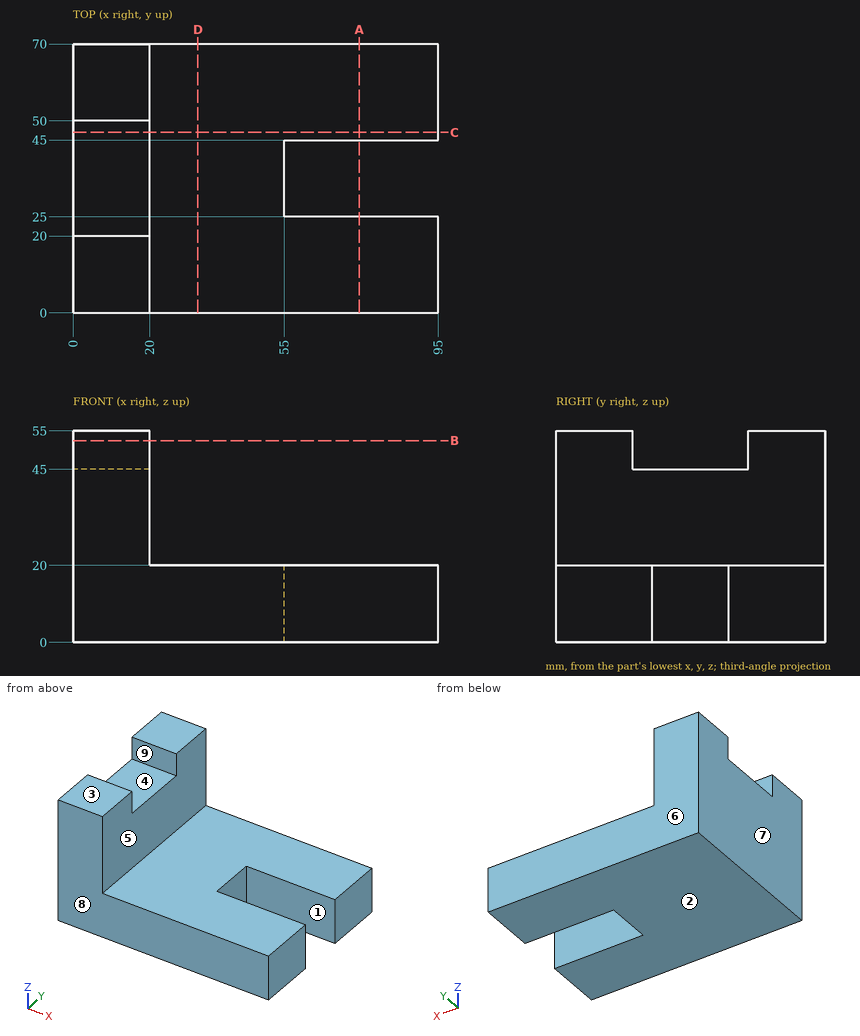
The drawing under review shows one solid part. Ordinate dimensions are in mm from its lowest x, y, z. A direction names the side the tool comes from. Coordinates: 2 decimals unless noted, no trailing zeros. Write each loop counter-clockwise with the first axis right and the second up, starting at its lowest first coordinate (ties: lowest second). Pieces come first, ordered by that corner, then holes. Notation, with made-up numbers: (46.5, 64) - (94.5, 64) arc R21 cw to (94.5, 98) - close; hole circle Ø3 at (73, 59). An arc over 180 degrees is marked (long way). Answer in a Markdown table with one row per item. Add a question column.
Q1. We need section D-D, the plane x = 32.5. State the section outline as (y, z) points.
Q2. Tool access review of the marked faces 1, 2, 3, 4 and 5: name each direction out of +Z, -Z, +X, -X, +Y, -Y from which nothing blocks a thin tool from reaching the whole face with its end or side.
Q3. We need section A-A, the plane x = 74.5. State the section outline as (y, z) points.
Q4. We need section B-B, the plane z = 52.5. State the section outline as (x, y) points, and give its area (3 significant figures).
Q5. Draft analysis for pull direction Y (two halves, no side actions). For the marked faces 6, 7, 8 and 9, state which applies: +Y half, -Y half, draft (parallel to the pull), parting line (faces both ways), or undercut.
Q6. For probe 1 along Y at (x, z) = (89, 17.5); probe 2 along Z at (x, y) = (18.5, 37); probe 3 along Z at (x, y) = (30, 58), list the stretches that pass through material, from the lowest coordinate up.
Q7. We need section C-C, the plane y = 47. State the section outline as (x, z) points.
Q8. For P1, Ø4, axis at x = 14.5, y = 27, coming from the +Z side; P2, Ø10, axis at y = 17.5, z = 28, coming from the +X side; P3, Ø10, axis at y = 38.5, z = 9, coming from the +X side, all flat-tipped, find the tip position at first contact; note any pin that passes through.
Answer list:
| question | item | result |
|---|---|---|
| 1 | outline | (0, 0) - (70, 0) - (70, 20) - (0, 20) - close |
| 2 | face 1 | +Z, -Z, +X |
| 2 | face 2 | -Z, +X, -X, +Y, -Y |
| 2 | face 3 | +Z, +X, -X, +Y, -Y |
| 2 | face 4 | +Z, +X, -X |
| 2 | face 5 | +Z, +X, +Y, -Y |
| 3 | outline | (0, 0) - (25, 0) - (25, 20) - (0, 20) - close; (45, 0) - (70, 0) - (70, 20) - (45, 20) - close |
| 4 | outline | (0, 0) - (20, 0) - (20, 20) - (0, 20) - close; (0, 50) - (20, 50) - (20, 70) - (0, 70) - close |
| 4 | area | 800 mm2 |
| 5 | face 6 | +Y half |
| 5 | face 7 | draft |
| 5 | face 8 | -Y half |
| 5 | face 9 | undercut |
| 6 | probe 1 | y = 0 to 25, 45 to 70 |
| 6 | probe 2 | z = 0 to 45 |
| 6 | probe 3 | z = 0 to 20 |
| 7 | outline | (0, 0) - (95, 0) - (95, 20) - (20, 20) - (20, 45) - (0, 45) - close |
| 8 | P1 | stops at z = 45 |
| 8 | P2 | stops at x = 20 |
| 8 | P3 | stops at x = 55 |
